Work out the finished part from the listing and answer in its coordinate system (mm). Face numbers are marked on the shaded views. Round coordinates to 2 decimals unless told otherwise and drop trailing zeros. Loops run counter-clockwise (first coordinate to the right, second up) from the corner with the lowest first, then second, coordinate; pieces in that order, holes last.
Autodesk Inventor part; units mm, degrees
ref_plane "LoftEndPlane" through (0, 0, 6) normal (0, 0, 1) x (1, 0, 0)
ref_plane "YZ Plane" through (0, 0, 0) normal (1, 0, 0) x (0, 1, 0)
ref_plane "XZ Plane" through (0, 0, 0) normal (0, 1, 0) x (-1, 0, 0)
sketch "Base" plane through (0, 0, 0) normal (0, 0, 1) x (1, 0, 0)
  circle A0 centre (0, 0) radius 8.5
  dimension "d0" = 17
extrude "BaseFeature" add sketch "Base" along normal blind 2
sketch "LoftStart" plane through (0, 0, 2) normal (0, 0, 1) x (1, 0, 0)
  circle A0 centre (0, 0) radius 8.5
ref_plane "LoftEndPlane" through (0, 0, 6) normal (0, 0, 1) x (1, 0, 0)
sketch "LoftEnd" plane through (0, 0, 6) normal (0, 0, 1) x (1, 0, 0)
  circle A0 centre (0, 0) radius 8.5 construction
  circle A1 centre (0, 0) radius 3
  dimension "d4" = 6
loft "BellLoftFeature" add profiles "LoftStart", "LoftEnd"
sketch "TopHole" plane through (0, 0, 6) normal (0, 0, 1) x (1, 0, 0)
  circle A0 centre (0, 0) radius 3
hole "TopHoleFeature" at (0, 0, 6) direction (0, 0, -1) diameter 3 end through all
properties part number "ForearmClampHead"
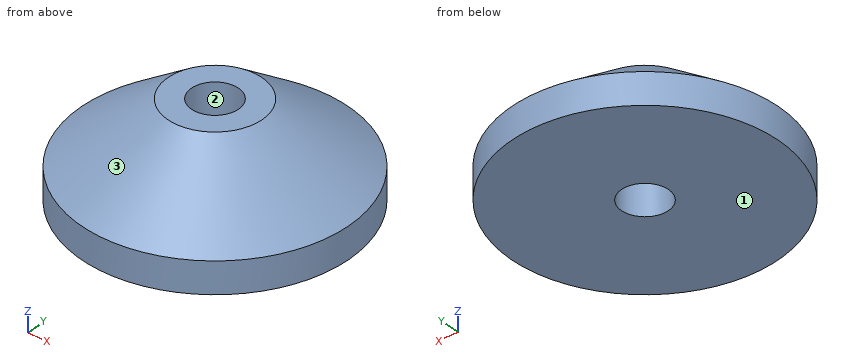
Item 1: Determine the mould class of the marked faces 1, 2 and 3 for opening direction X: pulls with the +X half, pulls with the -X half, needs draft (parallel to the pull), parting line crosses it, or undercut.
Item 2: Section C-C, the plane z = 5 is taken. Give the vertices of the cut face in (x, y) (3 decimals).
Item 3: Section A-A, the plane x = 0 is taken. Give the vertices of the cut face in (y, z), plus the area to 3 significant figures.
Item 4: Straight lines are drawn through the part: line 1 (Y direction, x = 0, z = 3.8) (3 decimals); line 2 (Y direction, x = 0, z = 3.4) (3 decimals); line 3 (X direction, y = 0.5, z = 3.25). For each, find the intervals that lie inside material, in ascending order.
Item 5: Section B-B, the plane z = 0.5 is taken. Give the vertices of the cut face in (x, y), plus the area to 3 significant figures.
Item 6: Each of these flat-tipped pins is pushed along its axis until it touches: P1, Ø1.5, axis at x = 4, z = 4, coming from the +Y side; P2, Ø1.5, axis at y = -3, z = 2, coming from the +X side; P3, Ø2, axis at y = -4.5, z = 0.5, coming from the -X side. Where does it stop, or does it pass through?
Answer below:
1. face 1: needs draft
1. face 2: undercut
1. face 3: parting line crosses it
2. outline: circle Ø8.75 at (0, 0); hole circle Ø3 at (0, 0)
3. outline: (-8.5, 0) - (-1.5, 0) - (-1.5, 6) - (-3, 6) - (-8.5, 2) - close; (1.5, 0) - (8.5, 0) - (8.5, 2) - (3, 6) - (1.5, 6) - close
3. area: 62.0 mm2
4. line 1: y = -6.025 to -1.5, 1.5 to 6.025
4. line 2: y = -6.575 to -1.5, 1.5 to 6.575
4. line 3: x = -6.76 to -1.41, 1.41 to 6.76
5. outline: circle Ø17 at (0, 0); hole circle Ø3 at (0, 0)
5. area: 220 mm2
6. P1: stops at y = 5.58
6. P2: stops at x = 8.2
6. P3: stops at x = -7.75
